For this review, take the finished solid that the model builds, in its own axes (mm). A direction names the side the tool comes from. Coordinates: 2 decimals unless noted, no trailing zeros. Order: outer loops, then holes, each group sorted by start corner. A loop starts at its lowest first (then second) coordinate and runs counter-clockwise, first axis right, second up. Notation, with made-up numbers: (29, 23.25) -> (80, 23.25) arc R21 ccw to (80, 50.25) -> close; hole circle Ø10 at (70, 71.25). An arc over 180 degrees is marked (long way). Return JSON: item names as keys, results as strings. Group by question number.
Item 1: Take a section at D-D (z = -2.6). Count the separate pieces of the cut face and the enclosed holes in it, then the cut area to 3 significant figures.
Item 2: Take a section at C-C (y = -3). Write out the cut boundary in (x, z) (3 decimals), then the cut area to 3 significant figures.
Item 3: Machinability: for faces 4 (the flat face through (161.069, -73.782, -1.565)), 5 (the flat face through (115.831, -107.766, -1.565)), 6 (the flat face through (34.04, -77.42, -1.57)), which of the approach directions +Z, -Z, +X, -X, +Y, -Y give a long, thin tool a straight path to every point of the face, cutting with its end or side? Answer none if there is none.
Item 4: Take a section at B-B (y = -94). Write out the cut boundary in (x, z) (3 decimals), then the cut area to 3 significant figures.
Item 5: Take a section at A-A (x = 87.63). Write out the cut boundary in (y, z) (3 decimals), then the cut area to 3 significant figures.
Item 6: Insertion check: pin 1 (1 mm diameter, centred on x = 32.5, z = -2.5, fed in from -Y); pin 2 (1.5 mm diameter, centred on y = -12, z = -0.5, fed in from +X); pin 3 (1 mm diameter, centred on y = -105, z = -2, fed in from -X). Each pin has a flat end and moves straight along its axis. Give the tip position at first contact, or say it passes through.
Item 7: Draft analysis for pull direction Y (two halves, no side actions). For faces 1 (the cylindrical face through (69.592, -66.536, -1.565)), 2 (the cylindrical face through (23.75, 1.45, -1.57)), 3 (the cylindrical face through (22.95, -14.38, -0.89)), state which applies: +Y half, -Y half, draft (parallel to the pull), parting line (faces both ways), or undercut.
Item 8: For line 1 along Y through (x, z) = (66.5, -2.75); line 2 along Y through (x, z) = (87.63, -2.15); line 3 along X through (y, z) = (-112, -2.9), list the stretches that pass through material, from the lowest coordinate up.
```python
from build123d import *

# Parameters (mm, degrees)
BOSS_EXTRUDE1_DEPTH                       = 3.175
F_6_CLEARANCE_HOLE1_D                     = 4.3053
SKETCH4_R                                 = 6.35
SKETCH4_R_2                               = 1.5875
SKETCH4_R_3                               = 4.7625
CUT_EXTRUDE1_DEPTH                        = 4.175
CSK_FOR_6_FLAT_HEAD_MACHINE_SCREW_2_COUNT = 2
CSK_FOR_6_FLAT_HEAD_MACHINE_SCREW_2_PITCH = 28.575
CSK_FOR_6_FLAT_HEAD_MACHINE_SCREW_3_COUNT = 2
CSK_FOR_6_FLAT_HEAD_MACHINE_SCREW_3_PITCH = 38.232062788
CSK_FOR_6_FLAT_HEAD_MACHINE_SCREW_4_COUNT = 2
CSK_FOR_6_FLAT_HEAD_MACHINE_SCREW_4_PITCH = 25.4
F_0_CLEARANCE_HOLE1_D                     = 1.8542
F_1_8_0_125_DIAMETER_HOLE1_D              = 3.175


with BuildPart() as part:
    # Sketch1 → Boss-Extrude1 (new body)
    with BuildSketch(Plane.XY):
        with BuildLine():
            Line((3.809986215, -91.884500325), (3.80998361, -115.403340545))
            ThreePointArc((3.80998361, -115.403340545), (3.999081622, -115.90576205), (4.472522544, -116.158821571))
            Line((4.472522544, -116.158821571), (38.023104274, -120.5758443))
            ThreePointArc((38.023104274, -120.5758443), (38.687459595, -120.33177166), (38.864463259, -119.646491316))
            Line((38.864463259, -119.646491316), (31.544635998, -88.413376307))
            ThreePointArc((31.544635998, -88.413376307), (31.412233483, -87.126289027), (31.609278422, -85.84750156))
            Line((31.609278422, -85.84750156), (36.533410401, -68.760772014))
            ThreePointArc((36.533410401, -68.760772014), (38.360231081, -66.108400459), (41.414754107, -65.0875))
            Line((41.414754107, -65.0875), (66.039990754, -65.0875))
            ThreePointArc((66.039990754, -65.0875), (69.632093202, -66.575397552), (71.119990754, -70.1675))
            Line((71.119990754, -70.1675), (71.119990754, -80.518))
            ThreePointArc((71.119990754, -80.518), (71.343175387, -81.056815367), (71.881990754, -81.28))
            Line((71.881990754, -81.28), (103.612235862, -81.28))
            ThreePointArc((103.612235862, -81.28), (106.604490402, -82.25478225), (108.448399818, -84.805034342))
            Line((108.448399818, -84.805034342), (123.423319929, -131.379161885))
            ThreePointArc((123.423319929, -131.379161885), (123.660593225, -131.731025839), (124.049283564, -131.901398021))
            Line((124.049283564, -131.901398021), (167.413526593, -137.610408921))
            ThreePointArc((167.413526593, -137.610408921), (168.015409063, -137.42782987), (168.274987552, -136.854927937))
            Line((168.274987552, -136.854927937), (168.274987552, -81.303553632))
            ThreePointArc((168.274987552, -81.303553632), (168.216983776, -81.011948907), (168.051802995, -80.764738341))
            Line((168.051802995, -80.764738341), (153.88788809, -66.600819412))
            ThreePointArc((153.88788809, -66.600819412), (152.786682817, -64.952748811), (152.399991049, -63.008717113))
            Line((152.399991049, -63.008717113), (152.399999892, -0.762021595))
            ThreePointArc((152.399999892, -0.762021595), (152.176815316, -0.223206231), (151.638, -2.1541e-05))
            Line((151.638, -2.1541e-05), (27.305, -3.804e-06))
            ThreePointArc((27.305, -3.804e-06), (23.712898123, 1.487894033), (22.22500087, 5.079996121))
            Line((22.22500087, 5.079996121), (22.225001755, 7.175496897))
            ThreePointArc((22.225001755, 7.175496897), (22.001816945, 7.7143128), (21.463001073, 7.937498421))
            Line((21.463001073, 7.937498421), (0.762001075, 7.937499892))
            ThreePointArc((0.762001075, 7.937499892), (0.223185691, 7.714315297), (1.021e-06, 7.175499945))
            Line((1.021e-06, 7.175499945), (-1.2342e-05, -87.949548922))
            ThreePointArc((-1.2342e-05, -87.949548922), (0.214550622, -88.479602508), (0.737406874, -88.711153328))
            ThreePointArc((0.737406874, -88.711153328), (2.915974038, -89.675944454), (3.809986215, -91.884500325))
        make_face()
    extrude(amount=-BOSS_EXTRUDE1_DEPTH)

    # #6 Clearance Hole1 (through all)
    with Locations(Plane(origin=(0, 0, -3.175), x_dir=(-1, 0, 0), z_dir=(0, 0, -1))):
        with Locations((-11.112500541, 3.81), (-18.414998872, -7.937503157), (-103.187497835, -15.240014658), (-143.510001128, -44.450020387), (-158.750001128, -111.125021649), (-18.414987678, -86.741003157), (-66.674991751, -58.7375), (-10.16, -110.502822935), (-146.049997068, -20.637520747), (-161.924987552, -130.483035149)):
            Hole(F_6_CLEARANCE_HOLE1_D / 2)

    # Sketch4 → Cut-Extrude1 (cut, through all)
    with BuildSketch(Plane(origin=(0, 0, -3.175), x_dir=(-1, 0, 0), z_dir=(0, 0, -1))):
        with Locations((-140.334987552, -115.57)):
            Circle(SKETCH4_R)
        with Locations((-124.205996572, -71.437521424)):
            Circle(SKETCH4_R)
        with Locations((-87.63, -62.992021649)):
            Circle(SKETCH4_R)
        with Locations((-87.63, -24.130021649)):
            Circle(SKETCH4_R)
        with Locations((-124.205996572, -24.130021649)):
            Circle(SKETCH4_R)
        with Locations((-124.205996572, -80.962521424)):
            Circle(SKETCH4_R_2)
        with Locations((-39.36999484, -36.322003157)):
            Circle(SKETCH4_R_3)
    extrude(amount=-CUT_EXTRUDE1_DEPTH, mode=Mode.SUBTRACT)

    # Sketch5 → CSK for #6 Flat Head Machine Screw (100)1 (revolve, cut)
    with BuildSketch(Plane(origin=(53.65749484, -14.097003157, -3.175), x_dir=(0, 1, 0), z_dir=(1, 0, 0))):
        Polygon((0, 0), (0, 3.175), (2.15265, 3.175), (2.15265, 1.420893136), (3.8460045, 0), align=None)
    csk_for_6_flat_head_machine_screw_100 = revolve(axis=Axis((53.65749484, -14.097003157, -9.525), (0, 0, 1)), mode=Mode.SUBTRACT)

    # CSK for _6 Flat Head Machine Screw _ 2: CSK for #6 Flat Head Machine Screw (100)1 ×2
    with Locations(*[(-i * CSK_FOR_6_FLAT_HEAD_MACHINE_SCREW_2_PITCH, 0, 0) for i in range(1, CSK_FOR_6_FLAT_HEAD_MACHINE_SCREW_2_COUNT)]):
        add(csk_for_6_flat_head_machine_screw_100, mode=Mode.SUBTRACT)

    # CSK for _6 Flat Head Machine Screw _ 3: CSK for #6 Flat Head Machine Screw (100)1 ×2
    with Locations(*[Vector(-0.747409319, -0.664363839, 0) * (i * CSK_FOR_6_FLAT_HEAD_MACHINE_SCREW_3_PITCH) for i in range(1, CSK_FOR_6_FLAT_HEAD_MACHINE_SCREW_3_COUNT)]):
        add(csk_for_6_flat_head_machine_screw_100, mode=Mode.SUBTRACT)

    # CSK for _6 Flat Head Machine Screw _ 4: CSK for #6 Flat Head Machine Screw (100)1 ×2
    with Locations(*[(0, -i * CSK_FOR_6_FLAT_HEAD_MACHINE_SCREW_4_PITCH, 0) for i in range(1, CSK_FOR_6_FLAT_HEAD_MACHINE_SCREW_4_COUNT)]):
        add(csk_for_6_flat_head_machine_screw_100, mode=Mode.SUBTRACT)

    # #0 Clearance Hole1 (through all)
    with Locations(Plane(origin=(0, 0, -9.525), x_dir=(-1, 0, 0), z_dir=(0, 0, -1))):
        with Locations((-39.36999484, -44.577003157)):
            Hole(F_0_CLEARANCE_HOLE1_D / 2)

    # 1/8 (0.125) Diameter Hole1 (through all)
    with Locations(Plane.XY):
        with Locations((39.36999484, -44.577003157)):
            Hole(F_1_8_0_125_DIAMETER_HOLE1_D / 2)


solid = part.part
```
Findings below:
{
 "1": {"separate pieces": "1", "enclosed holes": "22", "area": "15,100 mm2"},
 "2": {"outline": "(0, -3.175) -> (152.4, -3.175) -> (152.4, 0) -> (0, 0) -> close", "area": "484 mm2"},
 "3": {"face 4": "+Z, -Z, +X, +Y", "face 5": "+Z, -Z, -Y", "face 6": "+Z, -Z"},
 "4": {"outline": "(3.81, -3.175) -> (32.854, -3.175) -> (32.854, 0) -> (3.81, 0) -> close; (111.405, -3.175) -> (168.275, -3.175) -> (168.275, 0) -> (111.405, 0) -> close", "area": "273 mm2"},
 "5": {"outline": "(-81.28, -3.175) -> (-69.342, -3.175) -> (-69.342, 0) -> (-81.28, 0) -> close; (-56.642, -3.175) -> (-30.48, -3.175) -> (-30.48, 0) -> (-56.642, 0) -> close; (-17.78, -3.175) -> (0, -3.175) -> (0, 0) -> (-17.78, 0) -> close", "area": "177 mm2"},
 "6": {"pin 1": "stops at y = -119.91", "pin 2": "stops at x = 152.4", "pin 3": "stops at x = 3.81"},
 "7": {"face 1": "-Y half", "face 2": "+Y half", "face 3": "undercut"},
 "8": {"line 1": "y = -65.11 to -60.88, -56.59 to 0", "line 2": "y = -81.28 to -69.34, -56.64 to -30.48, -17.78 to 0", "line 3": "x = 3.81 to 8.61, 11.71 to 37.07, 117.19 to 135.08, 145.59 to 156.78, 160.72 to 168.27"}
}
